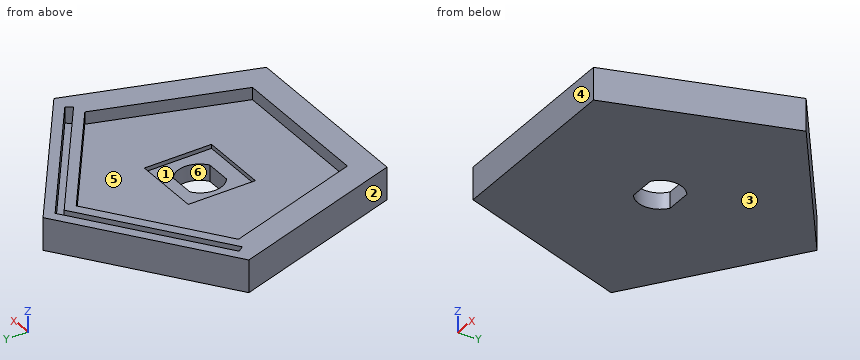
from build123d import *

# Parameters (mm, degrees)
PAD_DEPTH       = 8
POCKET_DEPTH    = 4
POCKET001_DEPTH = 3
POCKET002_DEPTH = 5
SKETCH004_W     = 16.5
SKETCH004_H     = 16.5
POCKET003_DEPTH = 1


with BuildPart() as part:
    # Sketch → Pad (new body)
    with BuildSketch(Plane.XY):
        Polygon((0, 38.536997), (-36.650862, 11.908587), (-22.651479, -31.177086), (22.651479, -31.177086), (36.650862, 11.908587), align=None)
    extrude(amount=PAD_DEPTH)

    # Sketch001 (on Face7 of Pad) → Pocket (cut)
    with BuildSketch(Plane.XY.offset(8)):
        Polygon((-32.77148, 11.76056), (0, 35.570434), (32.77148, 11.76056), (31.713466, 10.30433), (0, 33.345512), (-31.713466, 10.30433), align=None)
    extrude(amount=-POCKET_DEPTH, mode=Mode.SUBTRACT)

    # Sketch002 (on Face5 of Pocket) → Pocket001 (cut)
    with BuildSketch(Plane.XY.offset(8)):
        Polygon((0, 30.378949), (-28.892097, 9.387611), (-17.856298, -24.577086), (17.856298, -24.577086), (28.892097, 9.387611), align=None)
    extrude(amount=-POCKET001_DEPTH, mode=Mode.SUBTRACT)

    # Sketch003 (on Face20 of Pocket001) → Pocket002 (cut)
    with BuildSketch(Plane.XY.offset(5)):
        with BuildLine():
            ThreePointArc((-3.162278, 4.5), (-5.5, 0), (-3.162278, -4.5))
            Line((3.162278, -4.5), (-3.162278, -4.5))
            ThreePointArc((3.162278, -4.5), (5.5, 0), (3.162278, 4.5))
            Line((-3.162278, 4.5), (3.162278, 4.5))
        make_face()
    extrude(amount=-POCKET002_DEPTH, mode=Mode.SUBTRACT)

    # Sketch004 (on Face23 of Pocket002) → Pocket003 (cut)
    with BuildSketch(Plane.XY.offset(5)):
        Rectangle(SKETCH004_W, SKETCH004_H)
    extrude(amount=-POCKET003_DEPTH, mode=Mode.SUBTRACT)


solid = part.part
The model under review builds one solid part; all positions refer to its coordinate system, in mm. Face numbers are marked on the shaded views. A direction names the side the tool comes from. Round coordinates to 2 decimals unless told otherwise and drop trailing zeros. Loops run counter-clockwise (first coordinate to the right, second up) from the corner with the lowest first, then second, coordinate; pieces in that order, holes last. Notation, with made-up numbers: M 86,21 L 138,21 A20 cw 138,31 Z; hole C 50.25,24 d2. An arc over 180 degrees is marked long. Answer as CSV lines item,"result". Start each with the question number.
Item 1: Insertion check: P1, Ø2.5, axis at x = 2.5, z = 7, coming from the +Y side; P2, Ø7.5, axis at x = -6.5, y = 18.5, coming from the +Z side; P3, Ø1.1, axis at x = -3, z = 4.5, coming from the +Y side. Each pin has a flat end and moves straight along its axis. Give the tip position at first contact, or say it passes through.
Item 2: Consider section B-B (x = 1.5). Write out the cut boundary in (y, z).
Item 3: For the marked faces 4, 5 and 6, list the 3-axis set-ups (+Z, -Z, +X, -X, +Y, -Y) from which the entire face can be reached by the end or side of a thin tool; tool diameter is ignored.
Item 4: Mouldability with a two-part tool opening along X and no side actions: class the marked faces 1, 2 and 3 as released by +X, released by -X, zero draft, split by the parting line, or undercut.
Item 5: Consider section A-A (z = 6). Write out the cut boundary in (x, y), then the cut area to 3 significant figures.
Item 6: Consider section D-D (x = 19). Write out the cut boundary in (y, z).
Item 7: Wall thickness on line 1 (X direction, y = 15.5, z = 6.5); line 2 (X direction, y = 22, z = 5.75); line 3 (Z direction, x = 11, y = -4): over which ranges is each line inside the solid? List them lowest first. Write a range as [from, to].
Item 8: Consider section C-C (y = 3.5). Write out the cut boundary in (x, z).
Answer:
1,P1,"stops at y = 37.63"
1,P2,"stops at z = 5"
1,P3,"stops at y = 36.76"
2,outline,"M -31.18,0 L -4.5,0 L -4.5,4 L -8.25,4 L -8.25,5 L -24.58,5 L -24.58,8 L -31.18,8 Z; M 4.5,0 L 37.45,0 L 37.45,8 L 34.48,8 L 34.48,4 L 32.26,4 L 32.26,8 L 29.29,8 L 29.29,5 L 8.25,5 L 8.25,4 L 4.5,4 Z"
3,face 4,"+Z, -Z, +X, -X, -Y"
3,face 5,"+Z"
3,face 6,"+Z, -Z"
4,face 1,"undercut"
4,face 2,"released by -X"
4,face 3,"zero draft"
5,outline,"M -36.65,11.91 L -22.65,-31.18 L 22.65,-31.18 L 36.65,11.91 L 0,38.54 Z; hole M -32.77,11.76 L -31.71,10.3 L 0,33.35 L 31.71,10.3 L 32.77,11.76 L 0,35.57 Z; hole M -28.89,9.39 L -17.86,-24.58 L 17.86,-24.58 L 28.89,9.39 L 0,30.38 Z"
5,area,"1,190 mm^2"
6,outline,"M -31.18,0 L 24.73,0 L 24.73,8 L 21.77,8 L 21.77,4 L 19.54,4 L 19.54,8 L 16.57,8 L 16.57,5 L -21.06,5 L -21.06,8 L -31.18,8 Z"
7,line 1,"x = [-31.71, -27.62], [-24.56, -20.48], [20.48, 24.56], [27.62, 31.71]"
7,line 2,"x = [-22.76, -18.68], [-15.62, -11.53], [11.53, 15.62], [18.68, 22.76]"
7,line 3,"z = [0, 5]"
8,outline,"M -33.92,0 L -4.24,0 L -4.24,4 L -8.25,4 L -8.25,5 L -26.98,5 L -26.98,8 L -33.92,8 Z; M 4.24,0 L 33.92,0 L 33.92,8 L 26.98,8 L 26.98,5 L 8.25,5 L 8.25,4 L 4.24,4 Z"
